from build123d import *

# Parameters (mm, degrees)
BASE_FLANGE1_DEPTH      = 75
SKETCH4_R               = 20
CUT_EXTRUDE1_DEPTH      = 3
MITER_START             = 4
MITER_FLANGE1_DEPTH     = 76
MITER_FLANGE1_2_DEPTH   = 76
EDGE_FLANGE1_DEPTH      = 78
EDGE_FLANGE1_BEND_DEPTH = 32.152557442


# Read off the part's stored shape, not the designer's step: Miter Flange1
# Sheet-metal steps are written as plain solids
with BuildPart() as part:
    # Sketch1 → Base-Flange1 (new body)
    with BuildSketch(Plane.XY):
        with BuildLine():
            Line((-90, 80), (-90, 4))
            ThreePointArc((-90, 4), (-88.828427125, 1.171572875), (-86, 0))
            Line((-86, 0), (86, 0))
            ThreePointArc((86, 0), (88.828427125, 1.171572875), (90, 4))
            Line((90, 4), (90, 80))
            Line((90, 80), (87, 80))
            Line((87, 80), (87, 4))
            ThreePointArc((87, 4), (86.707106781, 3.292893219), (86, 3))
            Line((86, 3), (-86, 3))
            ThreePointArc((-86, 3), (-86.707106781, 3.292893219), (-87, 4))
            Line((-87, 4), (-87, 80))
            Line((-87, 80), (-90, 80))
        make_face()
    extrude(amount=BASE_FLANGE1_DEPTH)

    # Sketch4 → Cut-Extrude1 (cut)
    with BuildSketch(Plane(origin=(0, 3, 0), x_dir=(1, 0, 0), z_dir=(0, 1, 0))):
        Circle(SKETCH4_R)
    extrude(amount=-CUT_EXTRUDE1_DEPTH, mode=Mode.SUBTRACT)

    # Miter Flange1 outline → Miter Flange1 (cut)
    with BuildSketch(Plane(origin=(0, 0, 0), x_dir=(1, 0, 0), z_dir=(0, 1, 0)).offset(MITER_START)):
        with BuildLine():
            ThreePointArc((-90, -1), (-89.968118785, -0.49598283), (-89.872983346, 0))
            Line((-89.872983346, 0), (-90, 0))
            Line((-90, 0), (-90, -1))
        make_face()
    extrude(amount=MITER_FLANGE1_DEPTH, mode=Mode.SUBTRACT)

    # Miter Flange1 2 outline → Miter Flange1 2 (add)
    with BuildSketch(Plane(origin=(0, 0, 0), x_dir=(1, 0, 0), z_dir=(0, 1, 0)).offset(MITER_START)):
        with BuildLine():
            Line((-57, 10), (-57, 16))
            Line((-57, 16), (-60, 16))
            Line((-60, 16), (-60, 10))
            ThreePointArc((-60, 10), (-62.050252532, 5.050252532), (-67, 3))
            Line((-67, 3), (-86, 3))
            ThreePointArc((-86, 3), (-88.449489743, 2.16227766), (-89.872983346, 0))
            Line((-89.872983346, 0), (-87, 0))
            Line((-87, 0), (-87, -1))
            ThreePointArc((-87, -1), (-86.707106781, -0.292893219), (-86, 0))
            Line((-86, 0), (-67, 0))
            ThreePointArc((-67, 0), (-59.928932188, 2.928932188), (-57, 10))
        make_face()
    extrude(amount=MITER_FLANGE1_2_DEPTH)

    # Mirror1: part across plane


with BuildPart() as part_1:
    add(part.part)
    add(part.part.mirror(Plane(origin=(87, 4, 75), x_dir=(1, 0, 0), z_dir=(0, 0, 1))))

    # Edge-Flange1 section (across the edge) → Edge-Flange1 (add)
    with BuildSketch(Plane(origin=(90, 95, 36), x_dir=(0, -1, 0), z_dir=(0, 0, 1))):
        with BuildLine():
            Line((-3, 1), (-3, 30))
            Line((-3, 30), (0, 30))
            Line((0, 30), (0, 1))
            ThreePointArc((0, 1), (0.292893219, 0.292893219), (1, 0))
            Line((1, 0), (15, 0))
            Line((15, 0), (15, -3))
            Line((15, -3), (1, -3))
            ThreePointArc((1, -3), (-1.828427125, -1.828427125), (-3, 1))
        make_face()
    extrude(amount=EDGE_FLANGE1_DEPTH)

    # Edge-Flange1 section 2 (across the edge) → Edge-Flange1 bend (add)
    with BuildSketch(Plane(origin=(-90, 95, 99.006927285), x_dir=(0, -1, 0), z_dir=(0, 0, -1))):
        with BuildLine():
            Line((-3, 1), (-3, 30))
            Line((-3, 30), (0, 30))
            Line((0, 30), (0, 1))
            ThreePointArc((0, 1), (0.292893219, 0.292893219), (1, 0))
            Line((1, 0), (15, 0))
            Line((15, 0), (15, -3))
            Line((15, -3), (1, -3))
            ThreePointArc((1, -3), (-1.828427125, -1.828427125), (-3, 1))
        make_face()
    extrude(amount=EDGE_FLANGE1_BEND_DEPTH)


solid = part_1.part
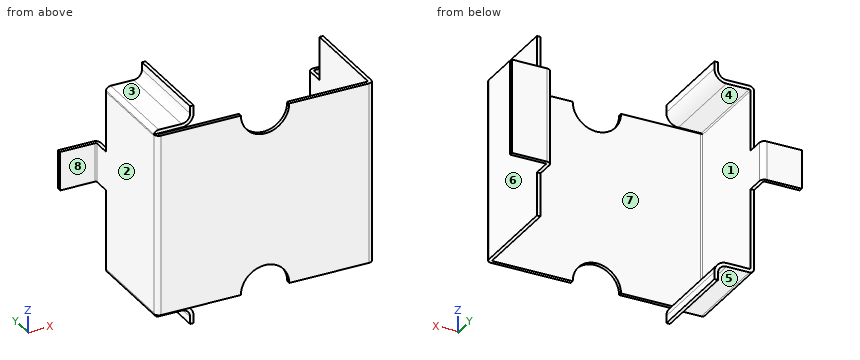
Geometry: final body of the model. Coordinates: model frame, mm. Face numbers are marked on the shaded views. A direction names the side the tool comes from. Coordinates: 2 decimals unless noted, no trailing zeros. Order: outer loops, then holes, each group sorted by start corner. A loop starts at its lowest first (then second) coordinate and runs counter-clockwise, first axis right, second up.
(1) Material intervals for probe 1 along X at (y, z) = (70.5, 49.5); probe 2 along Z at (x, y) = (-84.5, 21); probe 3 along Y at (x, z) = (-24.5, 83.5), sorted ascending.
(2) Section query B-B (z = 146). Return the cut outline in (x, y).
(3) Section query D-D (x = 31). Return the cut outline in (y, z).
(4) Draft query along Z for the marked faces 1, 2 and 3. Return one class per face: pulls with the +Z half, pulls with the -Z half, needs draft (parallel to the pull), parting line crosses it, or undercut.
(5) First-contact query: pin 1 (6.5 mm diameter, centred on y = 55, z = 163.5, fed in from -X); pin 2 (1.8 mm diameter, centred on y = 49, z = -14.5, fed in from +X); pin 3 (14.5 mm diameter, centred on x = -101.5, y = 88, fed in from -Z); pin 4 (18.5 mm diameter, centred on x = -67, z = 158, fed in from -Y). Flat tips, straight axial feed; report the tip coordinate or a pass-through.
(6) Access query for the marked faces 4, 5, 6, 7 and 8. Directions: +Z, -Z, +X, -X, +Y, -Y. A direction counts if a zero-diameter tool reaches every point of the face in a straight line with its end or side. Return the directions, or none.
(7) Section query A-A (y = 41.5). Return the cut outline in (x, z), plus the area to 3 significant figures.
(8) Section query C-C (z = 110.5). Return the cut outline in (x, y).
Solution:
1. probe 1: x = -90 to -87, 87 to 90
1. probe 2: z = -3 to 0, 150 to 153
1. probe 3: y = 0 to 3
2. outline: (-90, 4) arc R4 ccw to (-86, 0) - (-19.6, 0) - (-19.6, 3) - (-86, 3) arc R1 cw to (-87, 4) - (-87, 80) - (-90, 80) - close; (19.6, 0) - (86, 0) arc R4 ccw to (90, 4) - (90, 80) - (87, 80) - (87, 4) arc R1 cw to (86, 3) - (19.6, 3) - close
3. outline: (0, 0) - (3, 0) - (3, 150) - (0, 150) - close
4. face 1: undercut
4. face 2: needs draft
4. face 3: pulls with the +Z half
5. pin 1: stops at x = -60
5. pin 2: stops at x = -57
5. pin 3: stops at z = 66.85
5. pin 4: stops at y = 0
6. face 4: +Y
6. face 5: -Z, -X, +Y, -Y
6. face 6: +Z, -Z, +X, -Y
6. face 7: +Z, -Z, +Y
6. face 8: +Z, -Z, -X, -Y
7. outline: (-90, 1) arc R4 ccw to (-86, -3) - (-67, -3) arc R7 cw to (-60, -10) - (-60, -16) - (-57, -16) - (-57, -10) arc R10 ccw to (-67, 0) - (-86, 0) arc R1 cw to (-87, 1) - (-87, 149) arc R1 cw to (-86, 150) - (-67, 150) arc R10 ccw to (-57, 160) - (-57, 166) - (-60, 166) - (-60, 160) arc R7 cw to (-67, 153) - (-86, 153) arc R4 ccw to (-90, 149) - close; (87, 0) - (90, 0) - (90, 150) - (87, 150) - close
7. area: 1,150 mm2
8. outline: (-90, 4) arc R4 ccw to (-86, 0) - (86, 0) arc R4 ccw to (90, 4) - (90, 94) arc R1 cw to (91, 95) - (120, 95) - (120, 98) - (91, 98) arc R4 ccw to (87, 94) - (87, 4) arc R1 cw to (86, 3) - (-86, 3) arc R1 cw to (-87, 4) - (-87, 80) - (-90, 80) - close
